```python
from build123d import *

# Parameters (mm, degrees)
F0_R     = 6
F1_DEPTH = 25


with BuildPart() as f1:
    # F0 (on Front) → F1 (new body)
    with BuildSketch(Plane.XZ):
        with BuildLine():
            Line((26, -20), (34.641016, -20))
            ThreePointArc((34.641016, -20), (0, 40), (-34.641016, -20))
            Line((-34.641016, -20), (-23.449086, -20))
            Line((-23.449086, -20), (0, -20))
            ThreePointArc((0, -20), (2.12132, -19.12132), (3, -17))
            Line((3, -17), (3, 0))
            ThreePointArc((3, 0), (13, 10), (23, 0))
            Line((23, 0), (23, -17))
            ThreePointArc((23, -17), (23.87868, -19.12132), (26, -20))
        make_face()
        with Locations((-25, -6)):
            Circle(F0_R, mode=Mode.SUBTRACT)
    extrude(amount=F1_DEPTH)


solid = f1.part
```
Input: part model. Units: mm. Frame: model coordinates. A direction names the side the tool comes from. Coordinates: 2 decimals unless noted, no trailing zeros. Loops run counter-clockwise (first coordinate to the right, second up) from the corner with the lowest first, then second, coordinate; pieces in that order, holes last. Notation, with made-up numbers: (35.5, -26) - (83.5, -26) arc R22 ccw to (83.5, -11) - close; hole circle Ø1 at (-3.5, 3.25). An arc over 180 degrees is marked (long way). Answer in a Markdown table with one row per item.
(1) Material intervals for L1, parallel to X at y = -22, z = -4; L2, parallel to X at y = -7.5, z = -7.5; L3, parallel to X at y = -23, z = 4, sorted ascending. Write a range as from..to.
Model answer:
| item | result |
|---|---|
| L1 | x = -39.8..-30.66, -19.34..3, 23..39.8 |
| L2 | x = -39.29..-30.81, -19.19..3, 23..39.29 |
| L3 | x = -39.8..3.83, 22.17..39.8 |
(2) Cut plane A-A on y = -6. Output: boundary loops of the cut face in (x, z), plus the area to 3 significant figures.
Model answer:
| item | result |
|---|---|
| outline | (-34.64, -20) - (0, -20) arc R3 ccw to (3, -17) - (3, 0) arc R10 cw to (23, 0) - (23, -17) arc R3 ccw to (26, -20) - (34.64, -20) arc R40 ccw (long way) to start; hole circle Ø12 at (-25, -6) |
| area | 3,370 mm² |
(3) Cut plane B-B on z = -10. Output: boundary loops of the cut face in (x, y), plus the area to 3 significant figures.
Model answer:
| item | result |
|---|---|
| outline | (-38.73, -25) - (-29.47, -25) - (-29.47, 0) - (-38.73, 0) - close; (-20.53, -25) - (3, -25) - (3, 0) - (-20.53, 0) - close; (23, -25) - (38.73, -25) - (38.73, 0) - (23, 0) - close |
| area | 1,210 mm² |
(4) Mould query, pull axis X, two halves, no side actions, for faces 3 (the face through (-18, -12, -20)), 4 (the face through (3, -12, -9)), 5 (the face through (1.173, -12.325, 39.983)), 6 (the face through (23.86, -12.32, -19.1)). Classes: pulls with the +X half, pulls with the -X half, needs draft (parallel to the pull), parting line crosses it, or undercut.
Model answer:
| item | result |
|---|---|
| face 3 | needs draft |
| face 4 | undercut |
| face 5 | parting line crosses it |
| face 6 | undercut |
(5) Cut plane C-C on x = -22.5. Output: boundary loops of the cut face in (y, z).
Model answer:
| item | result |
|---|---|
| outline | (-25, -20) - (0, -20) - (0, -11.45) - (-25, -11.45) - close; (-25, -0.55) - (0, -0.55) - (0, 33.07) - (-25, 33.07) - close |
(6) Cut plane D-D on z = -3.5. Output: boundary loops of the cut face in (x, y).
Model answer:
| item | result |
|---|---|
| outline | (-39.85, -25) - (-30.45, -25) - (-30.45, 0) - (-39.85, 0) - close; (-19.55, -25) - (3, -25) - (3, 0) - (-19.55, 0) - close; (23, -25) - (39.85, -25) - (39.85, 0) - (23, 0) - close |
(7) Set-up query: faces 1 (the face through (-1, 0, 10)), 2 (the face through (23, -12, -8)). Return all of +Z, -Z, +X, -X, +Y, -Y with unobstructed straight access to the full face (end or side cutting, diameter ignored); none if empty.
Model answer:
| item | result |
|---|---|
| face 1 | +Z, -Z, +X, -X, +Y |
| face 2 | -Z, +Y, -Y |
(8) Pin query (flat end, axial travel): P1, Ø10, axis at y = -3.5, z = 31, coming from the +X side; P2, Ø5, axis at y = -15, z = -10.5, coming from the +X side; P3, Ø10, axis at y = -4.5, z = 2, coming from the -X side. Return the tip coordinate at first contact, or that it passes through.
Model answer:
| item | result |
|---|---|
| P1 | stops at x = 30.4 |
| P2 | stops at x = 39.19 |
| P3 | stops at x = -40 |
